The figure shows three views and two pictorial views of one solid part (mm, origin at its lowest corner). Answer the questions. A direction names the side the tool comes from. Coordinates: 2 decimals unless noted, no trailing zeros. Loops run counter-clockwise (first coordinate to the right, second up) from the corner with the lowest first, then second, coordinate; pieces in that order, holes last. Notation, with made-up numbers: (41, 58) - (97, 58) arc R18 ccw to (97, 74) - close; hole circle Ø7 at (41.5, 37.5). An arc over 180 degrees is marked (long way). Return JSON: item names as keys, results as strings. Group by question number.
1. Each of these flat-tipped pins is pushed along its axis until it touches: P1, Ø8, axis at x = 176, y = 237.5, coming from the +Z side (1 decimal); P2, Ø2, axis at y = 118, z = 108.5, coming from the +X side; P3, Ø1, axis at x = 120.5, y = 126, coming from the +Z side. Where does it stop, or does it pass through?
2. Section D-D (x = 129) is taken. Write down the section's boundary in (y, z).
3. Find the intervals of material crossed by line 1 along Z through (x, y) = (132.5, 129) (1 decimal); line 2 along Z through (x, y) = (103.5, 66.5); line 3 along Z through (x, y) = (251, 67) (1 decimal), in increasing order.
4. Which of the six approach directions +Z, -Z, +X, -X, +Y, -Y give full straight-line access (tool end or side, diameter ignored) to the marked faces 1, 2 and 3?
5. Section C-C (z = 119) is taken. Write down the section's boundary in (x, y) (1 decimal), and give its area (3 significant figures).
6. The mould has two halves that part along X. Classify the marked faces 4, 5 and 6: pulls with the +X half, pulls with the -X half, needs draft (parallel to the pull), parting line crosses it, or undercut.
7. Section B-B (x = 201) is taken. Write down the section's boundary in (y, z).
8. Section A-A (y = 33.5) is taken. Write down the section's boundary in (x, z) (1 decimal).
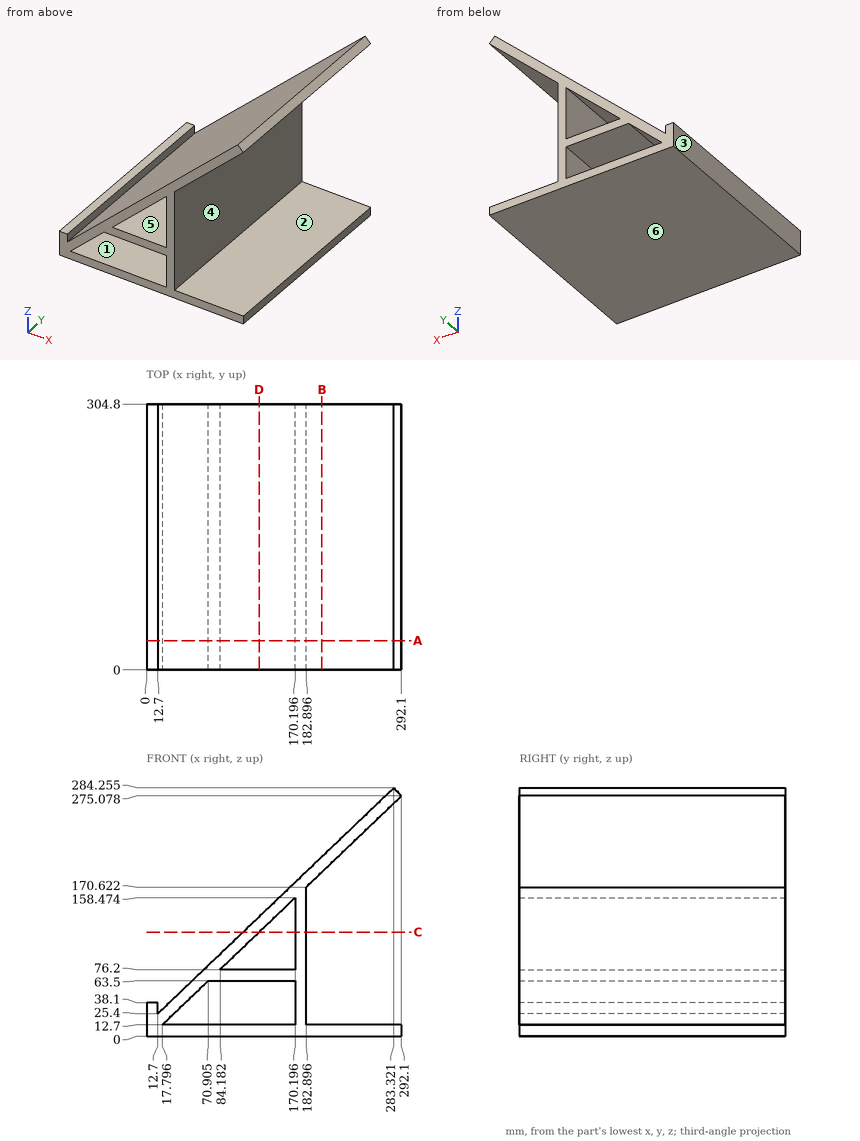
The answers:
{
 "1": {"P1": "stops at z = 185.4", "P2": "stops at x = 182.9", "P3": "stops at z = 128.99"},
 "2": {"outline": "(0, 0) - (304.8, 0) - (304.8, 12.7) - (0, 12.7) - close; (0, 63.5) - (304.8, 63.5) - (304.8, 76.2) - (0, 76.2) - close; (0, 119.07) - (304.8, 119.07) - (304.8, 136.64) - (0, 136.64) - close"},
 "3": {"line 1": "z = 0 to 12.7, 63.5 to 76.2, 122.4 to 140", "line 2": "z = 0 to 12.7, 63.5 to 76.2, 94.68 to 112.25", "line 3": "z = 0 to 12.7, 235.8 to 253.3"},
 "4": {"face 1": "+Y, -Y", "face 2": "+X, +Y, -Y", "face 3": "+Z, -Z, -X, +Y, -Y"},
 "5": {"outline": "(110.6, 0) - (128.9, 0) - (128.9, 304.8) - (110.6, 304.8) - close; (170.2, 0) - (182.9, 0) - (182.9, 304.8) - (170.2, 304.8) - close", "area": "9,470 mm2"},
 "6": {"face 4": "pulls with the +X half", "face 5": "undercut", "face 6": "needs draft"},
 "7": {"outline": "(0, 0) - (304.8, 0) - (304.8, 12.7) - (0, 12.7) - close; (0, 187.94) - (304.8, 187.94) - (304.8, 205.51) - (0, 205.51) - close"},
 "8": {"outline": "(0, 0) - (292.1, 0) - (292.1, 12.7) - (182.9, 12.7) - (182.9, 170.6) - (292.1, 275.1) - (283.3, 284.3) - (12.7, 25.4) - (12.7, 38.1) - (0, 38.1) - close; hole (17.8, 12.7) - (170.2, 12.7) - (170.2, 63.5) - (70.9, 63.5) - close; hole (84.2, 76.2) - (170.2, 76.2) - (170.2, 158.5) - close"}
}
